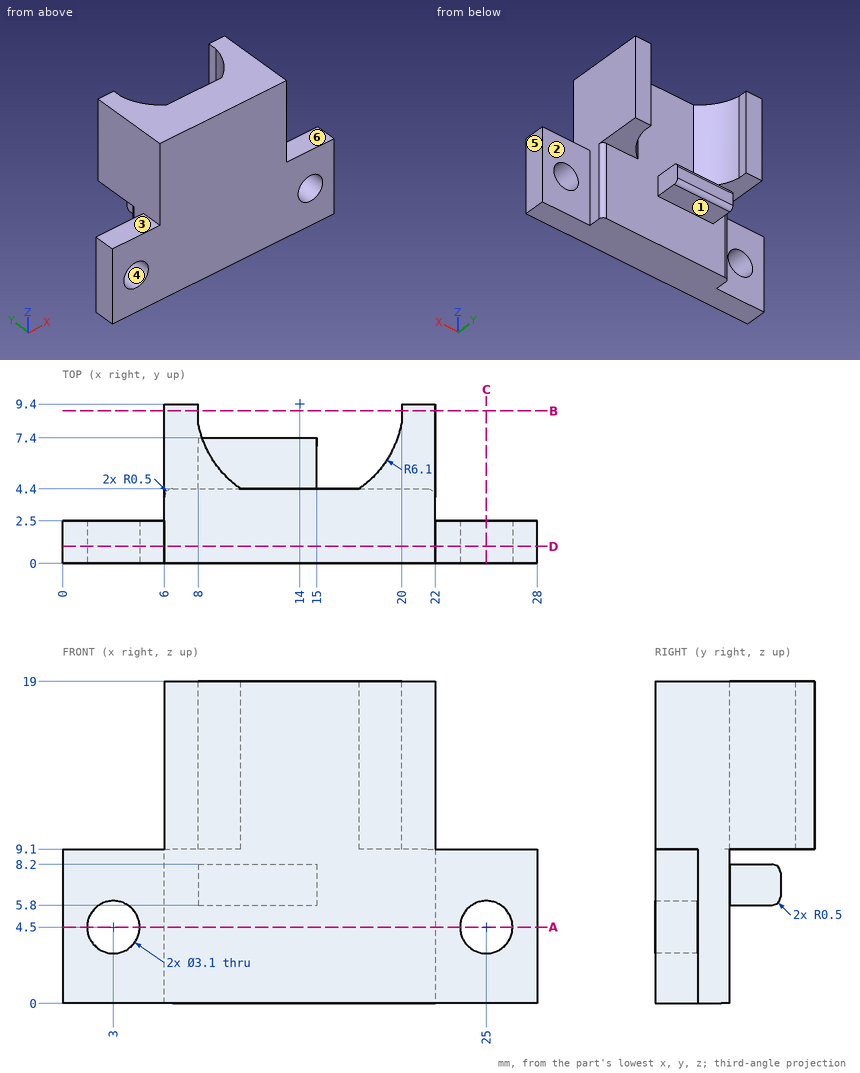
Source: three-view drawing plus pictorial views. Frame: mm from the lowest corner of the part. A direction names the side the tool comes from. Give positions to 0.01 mm unless a question says otherwise; leave off trailing zeros. Loops run counter-clockwise (first coordinate to the right, second up) from the corner with the lowest first, then second, coordinate; pieces in that order, holes last. Notation, with made-up numbers: (49.25, 38) -> (98.25, 38) arc R29 ccw to (98.25, 69) -> close; hole circle Ø7 at (46.25, 59.5). An arc over 180 degrees is marked (long way). Use a Markdown table: item, result. Add a question column.
(1) Pull-direction query (X, two-part tool) for the marked faces 4, 5 and 6; classes: +X half, -X half, draft (parallel to the pull), parting line (faces both ways), or undercut.
(2) Section query A-A (z = 4.5). Output: boundary loops of the cut face in (x, y).
(3) Section query C-C (x = 25). Output: boundary loops of the cut face in (y, z), then the cut area to 3 significant figures.
(4) Section query D-D (y = 1). Output: boundary loops of the cut face in (x, z).
(5) Section query B-B (y = 9). Output: boundary loops of the cut face in (x, z), then the cut area to 3 significant figures.
(6) Ray query, line 1 (X direction, y = 1.6, z = 4.5); line 2 (Z direction, x = 25, y = 0.75); line 3 (Y direction, x = 15, z = 16.75). Return the intervals inside material, ascending.
(7) Access query for the marked faces 1, 2 and 3. Directions: +Z, -Z, +X, -X, +Y, -Y. A direction counts if a zero-diameter tool reaches every point of the face in a straight line with its end or side. Return the directions, or none.
(8) First-contact query: pin 1 Ø7.5 at (x, z) = (14, 8) entering from +Y; pin 2 Ø2.5 at (y, z) = (6, 7.5) entering from -X; pin 3 Ø1.4 at (x, y) = (8.5, 5.5) entering from -Z; pin 4 Ø2 at (x, y) = (4, 3) entering from -Z. Flat tips, straight axial feed; report the tip coordinate or a pass-through.
Checked values:
| question | item | result |
|---|---|---|
| 1 | face 4 | undercut |
| 1 | face 5 | +X half |
| 1 | face 6 | draft |
| 2 | outline | (0, 0) -> (1.45, 0) -> (1.45, 2.5) -> (0, 2.5) -> close; (4.55, 0) -> (23.45, 0) -> (23.45, 2.5) -> (22, 2.5) -> (22, 3.9) arc R0.5 ccw to (21.5, 4.4) -> (6.5, 4.4) arc R0.5 ccw to (6, 3.9) -> (6, 2.5) -> (4.55, 2.5) -> close; (26.55, 0) -> (28, 0) -> (28, 2.5) -> (26.55, 2.5) -> close |
| 3 | outline | (0, 0) -> (2.5, 0) -> (2.5, 2.95) -> (0, 2.95) -> close; (0, 6.05) -> (2.5, 6.05) -> (2.5, 9.1) -> (0, 9.1) -> close |
| 3 | area | 15.0 mm^2 |
| 4 | outline | (0, 0) -> (28, 0) -> (28, 9.1) -> (22, 9.1) -> (22, 19) -> (6, 19) -> (6, 9.1) -> (0, 9.1) -> close; hole circle Ø3.1 at (3, 4.5); hole circle Ø3.1 at (25, 4.5) |
| 5 | outline | (6, 9.1) -> (8, 9.1) -> (8, 19) -> (6, 19) -> close; (20, 9.1) -> (22, 9.1) -> (22, 19) -> (20, 19) -> close |
| 5 | area | 39.6 mm^2 |
| 6 | line 1 | 0 to 1.45, 4.55 to 23.45, 26.55 to 28 |
| 6 | line 2 | 0 to 2.95, 6.05 to 9.1 |
| 6 | line 3 | 0 to 4.4 |
| 7 | face 1 | -Z, +X, -X, +Y |
| 7 | face 2 | +Z, -Z, +X, +Y |
| 7 | face 3 | +Z, -X, +Y, -Y |
| 8 | pin 1 | y = 7.4 |
| 8 | pin 2 | x = 8 |
| 8 | pin 3 | z = 5.8 |
| 8 | pin 4 | z = 0 |
